Autodesk Inventor part; units mm, degrees
ref_plane "YZ Plane" through (0, 0, 0) normal (1, 0, 0) x (0, 1, 0)
ref_plane "XZ Plane" through (0, 0, 0) normal (0, 1, 0) x (-1, 0, 0)
ref_plane "XY Plane" through (0, 0, 0) normal (0, 0, 1) x (1, 0, 0)
ref_plane "Work Plane1" through (0, 0, 2) normal (0, 0, 1) x (1, 0, 0)
sketch "Sketch1" plane through (0, 0, 2) normal (0, 0, 1) x (1, 0, 0)
  line L0 (-37.0712, 14) -> (-9.0712, 14) construction
  line L1 (-9.0712, 14) -> (-9.0712, -14) construction
  line L2 (-9.0712, -14) -> (-37.0712, -14) construction
  line L3 (-37.0712, -14) -> (-37.0712, 14) construction
  line L4 (-4.0712, -19) -> (-4.0712, 19)
  line L5 (-4.0712, 19) -> (-42.0712, 19)
  line L6 (-42.0712, 19) -> (-42.0712, -19)
  line L7 (-42.0712, -19) -> (-4.0712, -19)
  circle A0 centre (-23.0712, 0) radius 12.8
  point P0 (0, 0)
  dimension "d0" = 5
extrude "Extrusion1" add sketch "Sketch1" along normal blind 6 contours L7 L6 L5 L4 | A0
sketch "Sketch3" plane through (0, 0, 2) normal (0, 0, -1) x (-1, 0, 0)
  circle A0 centre (9.0712, -14) radius 1.45 construction
  circle A1 centre (9.0712, -14) radius 2.45
  circle A2 centre (37.0712, -14) radius 1.45
  circle A3 centre (37.0712, -14) radius 1.95
  point P0 (0, 0)
  dimension "d8" = 1
  dimension "d10" = 0.5
chamfer "Chamfer1" distance 3 angle 45 4 edges at (-42.0712, 19, 5) (-4.0712, 19, 5) (-4.0712, -19, 5) (-42.0712, -19, 5)
hole "Hole1" at (-37.0712, -14, 2) direction (0, 0, 1) diameter 4 depth 0.1 tip angle 100
sketch "Sketch4" plane through (-4.0712, -19, 2) normal (1, 0, 0) x (0, 0, -1)
  line L0 (2, 4.45) -> (6, 4.45)
  line L1 (2, 1.55) -> (6, 1.55)
  line L2 (0, 0) -> (0, 38)
  arc A0 (2, 19) -> (2, 19) centre (1.5, 4.4206) ccw
  line L3 (-1.7782, 5) -> (-0.1, 7)
  line L4 (-1.7782, 5) -> (-0.1, 3)
  line L5 (-0.1, 7) -> (0.6045, 7)
  line L6 (0.6045, 7) -> (0.6045, 3)
  line L7 (0.6045, 3) -> (-0.1, 3)
  line L8 (-0.1, 3) -> (-0.1, 7)
extrude "Extrusion4" cut sketch "Sketch4" against normal blind 8 contours L7 L8 L5 L2 | L2 L5 L6 L7 | L4 L3 L8
ref_plane "Arbeitsebene2" through (-23.0712, -12, 2) normal (1, 0, 0) x (0, 0, -1)
ref_plane "Arbeitsebene3" through (-39.0712, 0, 2) normal (0, -1, 0) x (1, 0, 0)
sketch "Skizze9" plane through (0, 0, 2) normal (0, 0, -1) x (-1, 0, 0)
  line L0 (12.0712, -16) -> (4.0712, -16)
  line L1 (7.0712, -19) -> (4.0712, -16)
  line L2 (39.0712, -19) -> (7.0712, -19)
  line L3 (42.0712, -16) -> (39.0712, -19)
  line L4 (42.0712, 16) -> (42.0712, -16)
  line L5 (39.0712, 19) -> (42.0712, 16)
  line L6 (7.0712, 19) -> (39.0712, 19)
  line L7 (4.0712, 16) -> (7.0712, 19)
  line L8 (4.0712, -12) -> (4.0712, 16)
  line L9 (4.0712, -12) -> (12.0712, -12)
  line L10 (12.0712, -12) -> (12.0712, -16)
  circle A0 centre (37.0712, -14) radius 2
  circle A1 centre (28.0712, -14) radius 3
  circle A2 centre (9.0712, 5) radius 3
  point P0 (0, 0)
  dimension "d54" = 6
  dimension "d55" = 6
  dimension "d56" = 14
  dimension "d57" = 5
  dimension "d58" = 5
  dimension "d59" = 14
extrude "Extrusion9" cut sketch "Skizze9" against normal blind 3 draft -2 contours A1 | A2
sketch "Skizze10" plane through (0, 0, 8) normal (0, 0, 1) x (1, 0, 0)
  circle A0 centre (-9.0712, 5) radius 4.05
  circle A1 centre (-28.0712, -14) radius 4.55
  circle A2 centre (-9.0712, 5) radius 4
  circle A3 centre (-28.0712, -14) radius 2.8952
  circle A4 centre (-28.0712, -14) radius 4
  point P0 (0, 0)
  dimension "d62" = 8
  dimension "d63" = 8
extrude "Extrusion10" cut sketch "Skizze10" against normal blind 5.5 contours A2 | A3 | A4
equation "\"d54\" = d55"
equation "\"d59\" = d56"
properties part number "20_Cube_Insert_Kinematic_Astromedia_30x40x1_45_pro_magnetic"
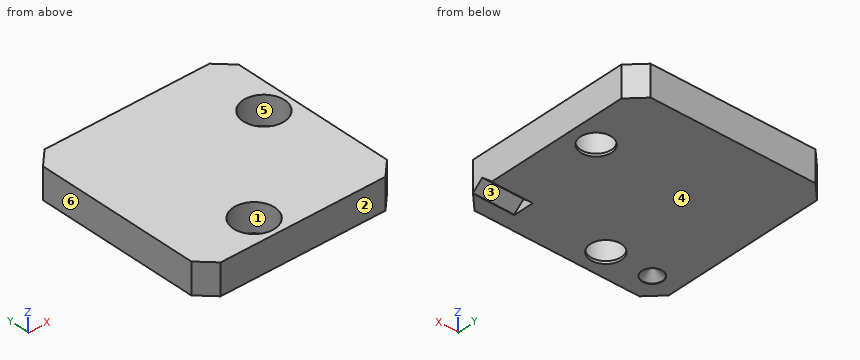
Read the model definition and answer for the solid it produces. Units are mm, in the model's axes. Face numbers are marked on the shaded views. A direction names the side the tool comes from. Round coordinates to 2 decimals unless told otherwise and drop trailing zeros. Write each loop counter-clockwise with the first axis right and the second up, starting at its lowest first coordinate (ties: lowest second). Pieces come first, ordered by that corner, then holes. Notation, with made-up numbers: (55.5, 37.5) -> (113.5, 37.5) arc R31 cw to (113.5, 75.5) -> close; hole circle Ø8 at (24.25, 15.5). An arc over 180 degrees is marked (long way). Answer in a Markdown table with one row per item. Add a question column.
1) Find section C-C, the plane z = 3.1. Determine the outline of the cut face in (x, y).
2) Find section B-B, the plane y = 5. Determine the outline of the cut face in (x, z), and give its area (3 significant figures).
3) Find section A-A, the plane z = 5.1. Determine the outline of the cut face in (x, y).
4) Consider line 1 (X direction, y = -14, z = 2.1); line 2 (Y direction, x = -11, z = 3); line 3 (Y direction, x = -28, z = 3.9). Determine where each line is inside the solid, lowest interval first.
5) Determine the mould class of the marked faces 1, 2, 3 and 4 for opening direction Y: pulls with the +Y half, pulls with the -Y half, needs draft (parallel to the pull), parting line crosses it, or undercut.
6) Given P1, Ø0.5, axis at y = -14, z = 2.5, coming from the +X side, flat-ended and moving along its own axis, determine where the tip first touches the part or whether it passes through.
7) Which of the six approach directions +Z, -Z, +X, -X, +Y, -Y give full straight-line access (tool end or side, diameter ignored) to the marked faces 5 and 6?
Findings below:
| question | item | result |
|---|---|---|
| 1 | outline | (-42.07, -16) -> (-39.07, -19) -> (-7.07, -19) -> (-4.07, -16) -> (-4.07, -14.81) -> (-12.07, -14.81) -> (-12.07, -13.19) -> (-4.07, -13.19) -> (-4.07, 16) -> (-7.07, 19) -> (-39.07, 19) -> (-42.07, 16) -> close; hole circle Ø1.62 at (-37.07, -14); hole circle Ø8 at (-28.07, -14); hole circle Ø8 at (-9.07, 5) |
| 2 | outline | (-42.07, 2) -> (-12.07, 2) -> (-12.05, 2.5) -> (-13.07, 2.5) -> (-13.07, 8) -> (-42.07, 8) -> close; (-6.09, 2.5) -> (-6.07, 2) -> (-4.07, 2) -> (-4.07, 8) -> (-5.07, 8) -> (-5.07, 2.5) -> close |
| 2 | area | 181 mm² |
| 3 | outline | (-42.07, -16) -> (-39.07, -19) -> (-7.07, -19) -> (-4.07, -16) -> (-4.07, 16) -> (-7.07, 19) -> (-39.07, 19) -> (-42.07, 16) -> close; hole circle Ø8 at (-28.07, -14); hole circle Ø8 at (-9.07, 5) |
| 4 | line 1 | -42.07 to -39.07, -35.07 to -31.07, -25.07 to -12.07 |
| 4 | line 2 | -19 to -14.93, -13.07 to 1.5, 8.5 to 19 |
| 4 | line 3 | -19 to -18, -10 to 19 |
| 5 | face 1 | undercut |
| 5 | face 2 | pulls with the -Y half |
| 5 | face 3 | undercut |
| 5 | face 4 | needs draft |
| 6 | P1 | x = -12.07 |
| 7 | face 5 | +Z |
| 7 | face 6 | +Z, -Z, -X, +Y, -Y |
